from build123d import *

# Parameters (mm, degrees)
F0_R     = 50.8
F0_R_2   = 44.45
F1_DEPTH = 152.4
F0_R_3   = 6.35
F2_DEPTH = 12.7
F3_R     = 6.35
F4_DEPTH = 63.5
F3_R_2   = 3.175
F5_DEPTH = 50.8010001


with BuildPart() as f1:
    # F0 (on Top) → F1 (new body)
    with BuildSketch(Plane.XY):
        Circle(F0_R)
        Circle(F0_R_2, mode=Mode.SUBTRACT)
    extrude(amount=F1_DEPTH)

    # F0 (on Top) → F2 (join)
    with BuildSketch(Plane.XY):
        Circle(F0_R)
        Circle(F0_R_2, mode=Mode.SUBTRACT)
        Circle(F0_R_2)
        Circle(F0_R_3, mode=Mode.SUBTRACT)
    extrude(amount=F2_DEPTH)

    # F3 (on Front) → F4 (cut, symmetric)
    with BuildSketch(Plane.XZ):
        with Locations((0, 127)):
            Circle(F3_R)
    extrude(amount=F4_DEPTH, both=True, mode=Mode.SUBTRACT)

    # F3 (on Front) → F5 (cut, through all)
    with BuildSketch(Plane.XZ):
        with Locations((0, 25.4)):
            Circle(F3_R_2)
    extrude(amount=F5_DEPTH, mode=Mode.SUBTRACT)


solid = f1.part
Check sheet for the modelled part. Datum: model origin and axes. Units: mm. A direction names the side the tool comes from. Round coordinates to 2 decimals unless told otherwise and drop trailing zeros. Order: outer loops, then holes, each group sorted by start corner. A loop starts at its lowest first (then second) coordinate and runs counter-clockwise, first axis right, second up.
(1) Cross-section at D-D, the plane x = -38. Enter the section's corners in (y, z), and give its area (3 significant figures).
(2) Go/stop test with flat-tipped pins: P1, Ø2, axis at x = 0.5, z = 82, coming from the -Y side; P2, Ø10, axis at x = 0, z = 127, coming from the -Y side; P3, Ø5, axis at y = -31, z = 44.5, coming from the -X side; P4, Ø5, axis at x = 0, z = 25.4, coming from the -Y side. Record where each tip stops, or that it passes through.
(3) Access from +Z, -Z, +X, -X, +Y, -Y to the whole of each face (thin tool, end or side, straight path). Record for faces 4 (the cylindrical face through (-0.41, -47.52, 28.55)), 5 (the cylindrical face through (-6.344, -47.449, 127.279)), 6 (the cylindrical face through (-9.6, -43.4, 81.6)).
(4) Draft check along X on faces 1 (the cylindrical face through (-1.38, -6.2, 6.26)), 2 (the flat face through (0, -45, 152.4)), 3 (the cylindrical face through (-11.012, -49.592, 75.133)). Enter one of: pulls with the +X half, pulls with the -X half, needs draft (parallel to the pull), parting line crosses it, or undercut.
(5) Cross-section at A-A, the plane x = 0. Enter the section's corners in (y, z) (3 decimals), and give its area (3 significant figures).
(6) Cross-section at C-C, the plane y = 40.5. Enter the section's corners in (x, z).
(7) Cross-section at B-B, the plane z = 127. Enter the section's corners in (x, y).
(8) Scan lines: probe 1 along Z at (x, y) = (0, -47.5) (3 decimals); probe 2 along Y at (x, z) = (0.5, 68.5); probe 3 along Y at (x, z) = (0, 9). Record each from-to range of solid material in increasing order.
Check sheet entries:
1. outline: (-33.71, 0) - (33.71, 0) - (33.71, 152.4) - (23.06, 152.4) - (23.06, 12.7) - (-23.06, 12.7) - (-23.06, 152.4) - (-33.71, 152.4) - close
1. area: 3,830 mm2
2. P1: stops at y = -50.8
2. P2: passes through
2. P3: stops at x = -42.05
2. P4: stops at y = 44.38
3. face 4: -Y
3. face 5: +Y, -Y
3. face 6: +Z
4. face 1: undercut
4. face 2: needs draft
4. face 3: parting line crosses it
5. outline: (-50.8, 0) - (-6.35, 0) - (-6.35, 12.7) - (-44.45, 12.7) - (-44.45, 22.225) - (-50.8, 22.225) - close; (-50.8, 28.575) - (-44.45, 28.575) - (-44.45, 120.65) - (-50.8, 120.65) - close; (-50.8, 133.35) - (-44.45, 133.35) - (-44.45, 152.4) - (-50.8, 152.4) - close; (6.35, 0) - (50.8, 0) - (50.8, 120.65) - (44.45, 120.65) - (44.45, 12.7) - (6.35, 12.7) - close; (44.45, 133.35) - (50.8, 133.35) - (50.8, 152.4) - (44.45, 152.4) - close
5. area: 2,700 mm2
6. outline: (-30.67, 0) - (30.67, 0) - (30.67, 152.4) - (18.32, 152.4) - (18.32, 12.7) - (-18.32, 12.7) - (-18.32, 152.4) - (-30.67, 152.4) - close
7. outline: (-6.35, -50.4) - (-6.35, -43.99) arc R44.45 cw to (-6.35, 43.99) - (-6.35, 50.4) arc R50.8 ccw to start; (6.35, -50.4) arc R50.8 ccw to (6.35, 50.4) - (6.35, 43.99) arc R44.45 cw to (6.35, -43.99) - close
8. probe 1: z = 0 to 22.225, 28.575 to 120.65, 133.35 to 152.4
8. probe 2: y = -50.8 to -44.45, 44.45 to 50.8
8. probe 3: y = -50.8 to -6.35, 6.35 to 50.8
